Model file for the job. Use its own axes, mm. Face numbers are marked on the shaded views. A direction names the side the tool comes from. Round coordinates to 2 decimals unless told otherwise and drop trailing zeros. Loops run counter-clockwise (first coordinate to the right, second up) from the corner with the lowest first, then second, coordinate; pieces in that order, holes last. Notation, with made-up numbers: (0.25, 23) - (39.25, 23) arc R11 ccw to (39.25, 39) - close; hole circle Ø7 at (36.5, 51). An arc over 180 degrees is marked (long way). Answer as a JSON object with one key per item and string values.
from build123d import *

# Parameters (mm, degrees)
BOSS_EXTRUDE1_DEPTH     = 100
CUT_EXTRUDE1_DEPTH      = 25
CUT_EXTRUDE1_DEPTH_BACK = 23


with BuildPart() as part:
    # Sketch1 → Boss-Extrude1 (new body)
    with BuildSketch(Plane(origin=(0, 0, 0), x_dir=(0, 0, -1), z_dir=(1, 0, 0))):
        with BuildLine():
            Line((-25.742274507, -27.603839777), (-25.742274507, -25.803839777))
            ThreePointArc((-25.742274507, -25.803839777), (-25.800853151, -25.66241842), (-25.942274507, -25.603839777))
            Line((-25.942274507, -25.603839777), (-26.659431795, -25.603839777))
            ThreePointArc((-26.659431795, -25.603839777), (-26.735968481, -25.588615683), (-26.800853151, -25.545261133))
            Line((-26.800853151, -25.545261133), (-27.683695863, -24.66241842))
            ThreePointArc((-27.683695863, -24.66241842), (-27.727050414, -24.597533751), (-27.742274507, -24.520997064))
            Line((-27.742274507, -24.520997064), (-27.742274507, -23.803839777))
            ThreePointArc((-27.742274507, -23.803839777), (-27.800853151, -23.66241842), (-27.942274507, -23.603839777))
            Line((-27.942274507, -23.603839777), (-28.659431795, -23.603839777))
            ThreePointArc((-28.659431795, -23.603839777), (-28.735968481, -23.588615683), (-28.800853151, -23.545261133))
            Line((-28.800853151, -23.545261133), (-29.683695863, -22.66241842))
            ThreePointArc((-29.683695863, -22.66241842), (-29.727050414, -22.597533751), (-29.742274507, -22.520997064))
            Line((-29.742274507, -22.520997064), (-29.742274507, -21.803839777))
            ThreePointArc((-29.742274507, -21.803839777), (-29.800853151, -21.66241842), (-29.942274507, -21.603839777))
            Line((-29.942274507, -21.603839777), (-30.659431795, -21.603839777))
            ThreePointArc((-30.659431795, -21.603839777), (-30.735968481, -21.588615683), (-30.800853151, -21.545261133))
            Line((-30.800853151, -21.545261133), (-31.683695863, -20.66241842))
            ThreePointArc((-31.683695863, -20.66241842), (-31.727050414, -20.597533751), (-31.742274507, -20.520997064))
            Line((-31.742274507, -20.520997064), (-31.742274507, -19.803839777))
            ThreePointArc((-31.742274507, -19.803839777), (-31.800853151, -19.66241842), (-31.942274507, -19.603839777))
            Line((-31.942274507, -19.603839777), (-32.659431795, -19.603839777))
            ThreePointArc((-32.659431795, -19.603839777), (-32.735968481, -19.588615683), (-32.800853151, -19.545261133))
            Line((-32.800853151, -19.545261133), (-33.683695863, -18.66241842))
            ThreePointArc((-33.683695863, -18.66241842), (-33.727050414, -18.597533751), (-33.742274507, -18.520997064))
            Line((-33.742274507, -18.520997064), (-33.742274507, -17.603839777))
            ThreePointArc((-33.742274507, -17.603839777), (-33.683695863, -17.46241842), (-33.542274507, -17.403839777))
            Line((-33.542274507, -17.403839777), (-23.442274507, -17.403839777))
            ThreePointArc((-23.442274507, -17.403839777), (-23.300853151, -17.46241842), (-23.242274507, -17.603839777))
            Line((-23.242274507, -17.603839777), (-23.242274507, -18.520997064))
            ThreePointArc((-23.242274507, -18.520997064), (-23.227050414, -18.597533751), (-23.183695863, -18.66241842))
            Line((-23.183695863, -18.66241842), (-22.300853151, -19.545261133))
            ThreePointArc((-22.300853151, -19.545261133), (-22.235968481, -19.588615683), (-22.159431795, -19.603839777))
            Line((-22.159431795, -19.603839777), (-21.442274507, -19.603839777))
            ThreePointArc((-21.442274507, -19.603839777), (-21.300853151, -19.66241842), (-21.242274507, -19.803839777))
            Line((-21.242274507, -19.803839777), (-21.242274507, -20.520997064))
            ThreePointArc((-21.242274507, -20.520997064), (-21.227050414, -20.597533751), (-21.183695863, -20.66241842))
            Line((-21.183695863, -20.66241842), (-20.300853151, -21.545261133))
            ThreePointArc((-20.300853151, -21.545261133), (-20.235968481, -21.588615683), (-20.159431795, -21.603839777))
            Line((-20.159431795, -21.603839777), (-19.442118142, -21.603839777))
            ThreePointArc((-19.442118142, -21.603839777), (-19.300696786, -21.66241842), (-19.242118142, -21.803839777))
            Line((-19.242118142, -21.803839777), (-19.242118142, -22.520623569))
            ThreePointArc((-19.242118142, -22.520623569), (-19.226894049, -22.597160256), (-19.183539499, -22.662044925))
            Line((-19.183539499, -22.662044925), (-18.242118142, -23.603466282))
            Line((-18.242118142, -23.603466282), (-17.742118142, -23.603466282))
            Line((-17.742118142, -23.603466282), (-13.499477455, -23.603466282))
            Line((-13.499477455, -23.603466282), (-21.035011361, -16.067932376))
            ThreePointArc((-21.035011361, -16.067932376), (-22.657128105, -14.984068619), (-24.570545267, -14.603466282))
            Line((-24.570545267, -14.603466282), (-25.960279372, -14.603466282))
            ThreePointArc((-25.960279372, -14.603466282), (-28.324188996, -13.859549098), (-29.658362326, -11.771137499))
            ThreePointArc((-29.658362326, -11.771137499), (-29.682182939, -11.531427852), (-29.647989066, -11.292976777))
            Line((-29.647989066, -11.292976777), (-26.628869488, -0.086805783))
            Line((-26.628869488, -0.086805783), (-28.360920296, -3.086805783))
            Line((-28.360920296, -3.086805783), (-41.233903642, -25.383466984))
            Line((-41.233903642, -25.383466984), (-42.615547882, -24.805037605))
            ThreePointArc((-42.615547882, -24.805037605), (-47.10930963, -14.877001433), (-37.531576616, -9.678268204))
            ThreePointArc((-37.531576616, -9.678268204), (-37.404269433, -9.668981846), (-37.308507446, -9.584583996))
            Line((-37.308507446, -9.584583996), (-32.078617814, -0.926149435))
            Line((-32.078617814, -0.926149435), (-45.393459966, -9.499644714))
            ThreePointArc((-45.393459966, -9.499644714), (-46.329728955, -10.180367196), (-47.181058303, -10.964727481))
            Line((-47.181058303, -10.964727481), (-47.811097829, -11.616550026))
            ThreePointArc((-47.811097829, -11.616550026), (-49.110536056, -13.39823645), (-49.874169518, -15.467006653))
            ThreePointArc((-49.874169518, -15.467006653), (-47.89514388, -23.874073774), (-40.105139668, -27.603839777))
            Line((-40.105139668, -27.603839777), (-25.742274507, -27.603839777))
        make_face()
    extrude(amount=BOSS_EXTRUDE1_DEPTH)

    # Sketch2 → Cut-Extrude1 (cut, two sides: drawn at the far end of the back side and taken through both)
    with BuildSketch(Plane(origin=(76.97885739, -34.993991596, 31.933978), x_dir=(1, 0, 0), z_dir=(0, 0, 1)).offset(-CUT_EXTRUDE1_DEPTH_BACK)):
        Polygon((-46.97885739, 36.842742805), (-6.97885739, 36.842742805), (-6.97885739, -2.226993345), (-46.97885739, -2.226993345), (-84.546864986, -2.226993345), (-84.546864986, 36.842742805), align=None)
    extrude(amount=CUT_EXTRUDE1_DEPTH + CUT_EXTRUDE1_DEPTH_BACK, mode=Mode.SUBTRACT)


solid = part.part
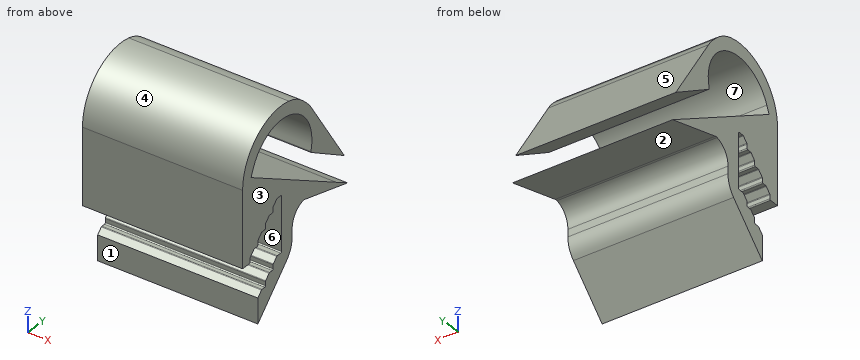
1) Slice it at B-B on y = -12.75. List the corners of the cut face in (x, z).
Values follow:
{"outline": "(70, 29.28) - (100, 29.28) - (100, 33.94) - (70, 33.94) - close; (70, 46.02) - (100, 46.02) - (100, 48.72) - (70, 48.72) - close"}
2) Probe probe 1 along Z at (x, y) = (82.75, -19.25); probe 2 along Y at (x, z) = (78, 26); probe 3 along Y at (x, z) = (95.75, 17.5). List the from-to ranges inside material, lowest first.
Values follow:
{"probe 1": "17.85 to 22.6, 33.1 to 37.69, 47.32 to 49.97", "probe 2": "-27.6 to -25.6, -17.4 to -14.6", "probe 3": "-23.6 to -19.6"}
3) Slice it at A-A on z = 42. List the corners of the cut face in (x, y), then the cut area to 3 significant figures.
Values follow:
{"outline": "(70, -27.42) - (100, -27.42) - (100, -25.06) - (70, -25.06) - close; (70, -9.82) - (100, -9.82) - (100, -7.31) - (70, -7.31) - close", "area": "146 mm²"}
4) Drop flat-ended pins along their axis: P1, Ø1.5, axis at x = 89, y = -13, coming from the +Z side; P2, Ø8, axis at x = 89.5, y = -12, coming from the -Z side; P3, Ø1.4, axis at x = 90, z = 15, coming from the -Y side. Give the stop position or say it passes through.
Values follow:
{"P1": "z = 49.29", "P2": "z = 21.1", "P3": "y = -23.6"}
5) Two-plate mould, pull along Y, no slides. Class the marked faces 4, 5, 6 and 7: pulls with the +Y half, pulls with the -Y half, needs draft (parallel to the pull), parting line crosses it, or undercut.
Values follow:
{"face 4": "parting line crosses it", "face 5": "pulls with the +Y half", "face 6": "undercut", "face 7": "undercut"}
6) Tool access for the marked faces 1, 2 and 3: list every direction of +Z, -Z, +X, -X, +Y, -Y with a clear straight run to the whole face (end or side of a thin tool).
Values follow:
{"face 1": "-Z, +X, -X, -Y", "face 2": "-Z, +X, -X", "face 3": "+Z, -Z, +X, +Y, -Y"}
